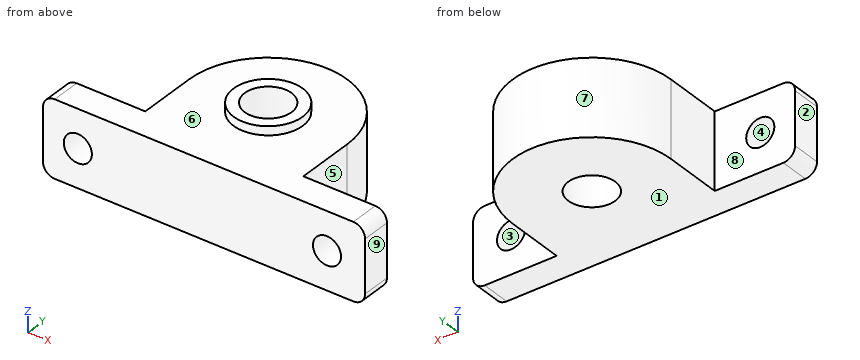
```python
from build123d import *

# Parameters (mm, degrees)
SKETCH2_R           = 4
BOSS_EXTRUDE1_DEPTH = 13
SKETCH3_R           = 5.9
SKETCH3_R_2         = 4
BOSS_EXTRUDE2_DEPTH = 1.5
SKETCH4_R           = 2.4
CUT_EXTRUDE1_DEPTH  = 5
FILLET1_R           = 2
FILLET2_R           = 2


with BuildPart() as part:
    # Sketch2 → Boss-Extrude1 (new body)
    with BuildSketch(Plane.XY):
        with BuildLine():
            Line((0, 0), (55, 0))
            Line((55, 0), (55, 5))
            Line((55, 5), (40.722217225, 5))
            Line((40.722217225, 5), (40.722217225, 15))
            ThreePointArc((40.722217225, 15), (27.222217225, 28.5), (13.722217225, 15))
            Line((13.722217225, 15), (13.722217225, 5))
            Line((13.722217225, 5), (0, 5))
            Line((0, 5), (0, 0))
        make_face()
        with Locations(Location((27.222217225, 15, 0), (0, 0, 180))):
            Circle(SKETCH2_R, mode=Mode.SUBTRACT)
    extrude(amount=BOSS_EXTRUDE1_DEPTH)

    # Sketch3 → Boss-Extrude2 (add)
    with BuildSketch(Plane.XY.offset(13)):
        with Locations((27.222217225, 15)):
            Circle(SKETCH3_R)
        with Locations(Location((27.222217225, 15, 0), (0, 0, 180))):
            Circle(SKETCH3_R_2, mode=Mode.SUBTRACT)
    extrude(amount=BOSS_EXTRUDE2_DEPTH)

    # Sketch4 → Cut-Extrude1 (cut)
    with BuildSketch(Plane(origin=(0, 5, 0), x_dir=(1, 0, 0), z_dir=(0, 1, 0))):
        with Locations(Location((48.5, -6.5, 0), (0, 0, 180))):
            Circle(SKETCH4_R)
        with Locations((5.944434451, -6.5)):
            Circle(SKETCH4_R)
    extrude(amount=-CUT_EXTRUDE1_DEPTH, mode=Mode.SUBTRACT)

    # Fillet1
    fillet1_edges = [part.edges().sort_by_distance(p)[0] for p in [
        (55, 2.5, 13),
    ]]
    fillet(fillet1_edges, radius=FILLET1_R)

    # Fillet2
    fillet2_edges = [part.edges().sort_by_distance(p)[0] for p in [
        (0, 2.5, 0),
        (0, 2.5, 13),
        (55, 2.5, 0),
    ]]
    fillet(fillet2_edges, radius=FILLET2_R)


solid = part.part
```
Source: CAD feature listing. Evaluate the final solid. Frame: model axes, mm. Face numbers are marked on the shaded views. A direction names the side the tool comes from. Give positions to 0.01 mm unless a question says otherwise; leave off trailing zeros. Write each loop counter-clockwise with the first axis right and the second up, starting at its lowest first coordinate (ties: lowest second). Pieces come first, ordered by that corner, then holes. Notation, with made-up numbers: (-11.75, 64) - (11.25, 64) arc R8 cw to (11.25, 75) - close; hole circle Ø11 at (-38, -8.75). An arc over 180 degrees is marked (long way). One line per item, written item: value. Start each with the question number.
Q1. Section query A-A, the plane x = 48.5. Return the cut outline in (y, z).
Q2. Draft query along Z for the marked faces 1, 2, 3 and 4. Return one class per face: +Z half, -Z half, draft (parallel to the pull), parting line (faces both ways), or undercut.
Q3. Material intervals for probe 1 along Z at (x, y) = (48.5, 2.4); probe 2 along X at (y, z) = (15.25, 12.5); probe 3 along Z at (x, y) = (15, 16.25), sorted ascending. Write a range as from..to.
Q4. Section query B-B, the plane z = 6.5. Return the cut outline in (x, y), then the cut area to 3 significant figures.
Q5. Section query C-C, the plane y = 13.75. Return the cut outline in (x, z).
Q6. First-contact query: pin 1 Ø5.5 at (x, z) = (48.5, 6.5) entering from -Y; pin 2 Ø4 at (x, z) = (45, 9) entering from +Y; pin 3 Ø8 at (y, z) = (10, 8) entering from +X; pin 4 Ø1 at (y, z) = (14.5, 12.5) entering from -X. Flat tips, straight axial feed; report the tip coordinate or a pass-through.
Q7. Section query D-D, the plane z = 9.5. Return the cut outline in (x, y), then the cut area to 3 significant figures.
Q8. Set-up query: the marked faces 5, 6, 7, 8 and 9. Return all of +Z, -Z, +X, -X, +Y, -Y with unobstructed straight access to the full face (end or side cutting, diameter ignored); none if empty.
Answer:
1. outline: (0, 0) - (5, 0) - (5, 4.1) - (0, 4.1) - close; (0, 8.9) - (5, 8.9) - (5, 13) - (0, 13) - close
2. face 1: -Z half
2. face 2: draft
2. face 3: undercut
2. face 4: undercut
3. probe 1: z = 0..4.1, 8.9..13
3. probe 2: x = 13.72..23.23, 31.21..40.72
3. probe 3: z = 0..13
4. outline: (0, 0) - (3.54, 0) - (3.54, 5) - (0, 5) - close; (8.34, 0) - (46.1, 0) - (46.1, 5) - (40.72, 5) - (40.72, 15) arc R13.5 ccw to (13.72, 15) - (13.72, 5) - (8.34, 5) - close; (50.9, 0) - (55, 0) - (55, 5) - (50.9, 5) - close; hole circle Ø8 at (27.22, 15)
4. area: 733 mm2
5. outline: (13.72, 0) - (23.42, 0) - (23.42, 14.5) - (21.46, 14.5) - (21.46, 13) - (13.72, 13) - close; (31.02, 0) - (40.72, 0) - (40.72, 13) - (32.99, 13) - (32.99, 14.5) - (31.02, 14.5) - close
6. pin 1: stops at y = 0
6. pin 2: stops at y = 5
6. pin 3: stops at x = 40.72
6. pin 4: stops at x = 13.72
7. outline: (0, 0) - (55, 0) - (55, 5) - (40.72, 5) - (40.72, 15) arc R13.5 ccw to (13.72, 15) - (13.72, 5) - (0, 5) - close; hole circle Ø8 at (27.22, 15)
7. area: 781 mm2
8. face 5: +Z, -Z, +X, +Y
8. face 6: +Z
8. face 7: +Z, -Z, +Y
8. face 8: +Z, -Z, -X, +Y
8. face 9: +Z, -Z, +X, +Y, -Y
